Autodesk Inventor part; units mm, degrees
ref_plane "YZ Plane" through (0, 0, 0) normal (1, 0, 0) x (0, 1, 0)
ref_plane "XZ Plane" through (0, 0, 0) normal (0, 1, 0) x (-1, 0, 0)
ref_plane "XY Plane" through (0, 0, 0) normal (0, 0, 1) x (1, 0, 0)
sketch "Sketch1" plane through (0, 0, 0) normal (0, 1, 0) x (-1, 0, 0)
  line L0 (-27.3558, 45.72) -> (27.3558, 45.72)
  line L1 (27.3558, 45.72) -> (27.3558, -45.72)
  line L2 (27.3558, -45.72) -> (-27.3558, -45.72)
  line L3 (-27.3558, -45.72) -> (-27.3558, 45.72)
  line L4 (-27.3558, 45.72) -> (27.3558, -45.72) construction
  line L5 (27.3558, 45.72) -> (-27.3558, -45.72) construction
  point P0 (0, 0)
  dimension "d0" = 54.7116
  dimension "d1" = 91.44
extrude "Extrusion1" add sketch "Sketch1" along normal blind 2.794
sketch "Sketch2" plane through (0, 2.794, 0) normal (0, 1, 0) x (1, 0, 0)
  circle A0 centre (-6.3442, 0) radius 6 construction
  circle A1 centre (0.6558, 0) radius 18.4 construction
  circle A2 centre (-7.0942, -13.4234) radius 1.25 construction
  circle A3 centre (-12.7676, -7.75) radius 1.25 construction
  circle A4 centre (-12.7676, 7.75) radius 1.25 construction
  circle A5 centre (-7.0942, 13.4234) radius 1.25 construction
  circle A6 centre (0.6558, 15.5) radius 1.25 construction
  circle A7 centre (14.0792, 7.75) radius 1.25 construction
  circle A8 centre (16.1558, 0) radius 1.25 construction
  circle A9 centre (14.0792, -7.75) radius 1.25 construction
  circle A10 centre (0.6558, -15.5) radius 1.25 construction
  spline S0 degree 3 poles (-6.3442, -8.58) (-7.0027, -8.6329) (-7.0027, -9.0013) (-6.3442, -9.6852) knots -1 -1 -1 -1 0 0 0 0 construction
  arc A11 (-6.3442, -9.6852) -> (-6.3442, 9.6852) centre (0.6558, 0) ccw construction
  spline S1 degree 3 poles (-6.3442, 9.6852) (-7.0027, 9.0013) (-7.0027, 8.6329) (-6.3442, 8.58) knots -1 -1 -1 -1 0 0 0 0 construction
  arc A12 (-6.3442, -8.58) -> (-6.3442, 8.58) centre (-6.3442, 0) ccw construction
  circle A13 centre (-6.3442, 0) radius 6.223
  point P0 (0, 0)
  dimension "d4" = 12.446
hole "Hole1" at (0.6558, 2.794, -15.5) at (0.6558, 2.794, 15.5) at (14.0792, 2.794, -7.75) at (14.0792, 2.794, 7.75) at (-12.7676, 2.794, -7.75) at (-12.7676, 2.794, 7.75) direction (0, -1, 0) diameter 3 end through all
extrude "Extrusion2" cut sketch "Sketch2" against normal blind 25.4
sketch "Sketch3" plane through (0, 2.794, 0) normal (0, 1, 0) x (1, 0, 0)
  point P0 (0, 0)
sketch "Sketch4" plane through (0, 0, 0) normal (0, -1, 0) x (1, 0, 0)
  arc A0 (8.0816, -16.5469) -> (10.5912, -15.0645) centre (9.1558, -15.5) ccw
  arc A1 (10.5912, -15.0645) -> (10.5912, 15.0645) centre (0, 0) ccw
  arc A2 (10.5912, 15.0645) -> (8.0816, 16.5469) centre (9.1558, 15.5) ccw
  arc A3 (8.0816, 16.5469) -> (8.0816, -16.5469) centre (0, 0) ccw
  circle A4 centre (-21.8442, -15.5) radius 1.5
  circle A5 centre (-21.8442, 15.5) radius 1.5
  arc A6 (-27.3558, -42.545) -> (-24.1808, -45.72) centre (-24.1808, -42.545) ccw
  line L0 (-27.3558, -42.545) -> (-27.3558, 42.545)
  arc A7 (-24.1808, 45.72) -> (-27.3558, 42.545) centre (-24.1808, 42.545) ccw
  line L1 (-24.1808, 45.72) -> (24.1808, 45.72)
  arc A8 (27.3558, 42.545) -> (24.1808, 45.72) centre (24.1808, 42.545) ccw
  line L2 (27.3558, 42.545) -> (27.3558, -42.545)
  arc A9 (24.1808, -45.72) -> (27.3558, -42.545) centre (24.1808, -42.545) ccw
  line L3 (24.1808, -45.72) -> (-24.1808, -45.72)
  circle A10 centre (9.1558, -15.5) radius 3.25
  circle A11 centre (9.1558, 15.5) radius 3.25
  point P0 (0, 0)
  dimension "d14" = 6.5
  dimension "d15" = 6.5
extrude "Extrusion3" cut sketch "Sketch4" against normal blind 25.4 contours A3 A10 A1 A0 | A0 A1 A10 A3 | A11 A1 A2 A3 | A3 A2 A1 A11 | A4 | A5
fillet "Fillet1" radius 3.175 4 edges at (-27.3558, 1.397, -45.72) (-27.3558, 1.397, 45.72) (27.3558, 1.397, 45.72) (27.3558, 1.397, -45.72)
equation "\"d15\" = d14"
properties part number "MotorMountDCB" material "Polycarbonate, Smoke"
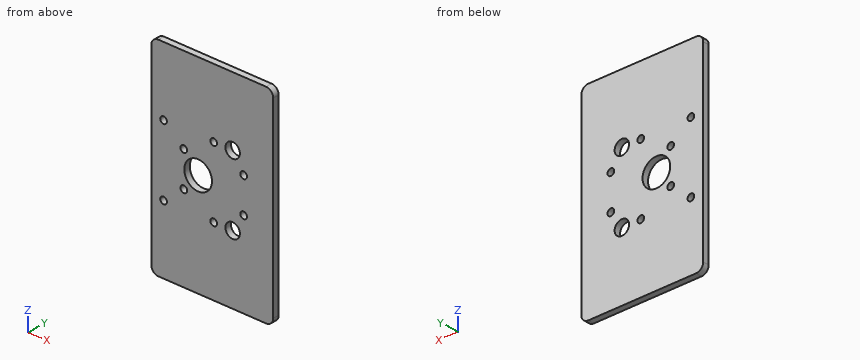
Geometry check sheet. Reference: the model listing, model coordinates, mm. Give positions to 0.01 mm unless a question says otherwise; leave off trailing zeros. Order: outer loops, then holes, each group sorted by start corner. A loop starts at its lowest first (then second) coordinate and runs counter-clockwise, first axis right, second up. Notation, with made-up numbers: (14, -6) - (64, -6) arc R16 ccw to (64, 6) - close; hole circle Ø9 at (-19.5, 57). An arc over 180 degrees is marked (long way). Use one line per item in the form item = value.
1) Sectioned sample at B-B (z = 15.5). Record the boundary of the cut face in (x, y), and give its area (3 significant figures).
Working result:
outline = (-27.36, 0) - (-23.34, 0) - (-23.34, 2.79) - (-27.36, 2.79) - close; (-20.34, 0) - (-0.84, 0) - (-0.84, 2.79) - (-20.34, 2.79) - close; (2.16, 0) - (5.91, 0) - (5.91, 2.79) - (2.16, 2.79) - close; (12.41, 0) - (27.36, 0) - (27.36, 2.79) - (12.41, 2.79) - close
area = 118 mm^2
2) Sectioned sample at A-A (z = 0). Record the boundary of the cut face in (x, y), and give its area (3 significant figures).
Working result:
outline = (-27.36, 0) - (-12.57, 0) - (-12.57, 2.79) - (-27.36, 2.79) - close; (-0.12, 0) - (27.36, 0) - (27.36, 2.79) - (-0.12, 2.79) - close
area = 118 mm^2
3) Sectioned sample at C-C (y = 1.85). Count the separate pieces of the cut face and the enclosed holes in it, and give its area (3 significant figures).
Working result:
separate_pieces = 1
enclosed_holes = 11
area = 4,750 mm^2
4) Material ranges on probe 1 along X at (y, z) = (1.3, 7.75); probe 2 along Z at (x, y) = (13, 1.3); probe 3 along Z at (x, y) = (8.5, 2.35), recorded low to high. Write a range as from..to.
Working result:
probe_1 = -27.36..-14.27, -11.27..12.58, 15.58..27.36
probe_2 = -45.72..-8.79, -6.71..6.71, 8.79..45.72
probe_3 = -45.72..-18.68, -12.32..12.32, 18.68..45.72
